from build123d import *

# Parameters (mm, degrees)
SKETCH1_R               = 8.895
BOSS_EXTRUDE1_DEPTH     = 25
CUT_EXTRUDE1_DEPTH      = 12.5
SKETCH3_R               = 1.984375
CUT_EXTRUDE2_DEPTH      = 9.895
CUT_EXTRUDE2_DEPTH_BACK = 9.895
CHAMFER1_SIZE           = 0.6


with BuildPart() as part:
    # Sketch1 → Boss-Extrude1 (new body)
    with BuildSketch(Plane(origin=(0, 0, 0), x_dir=(1, 0, 0), z_dir=(0, 1, 0))):
        Circle(SKETCH1_R)
    extrude(amount=-BOSS_EXTRUDE1_DEPTH)

    # Sketch2 → Cut-Extrude1 (cut)
    with BuildSketch(Plane.XZ.offset(25)):
        with BuildLine():
            Line((-6.83125, 1.984375), (-6.83125, -1.984375))
            Line((-6.83125, -1.984375), (-8.670829306, -1.984375))
            ThreePointArc((-8.670829306, -1.984375), (-8.895, 0), (-8.670829306, 1.984375))
            Line((-8.670829306, 1.984375), (-6.83125, 1.984375))
        make_face()
    cut_extrude1 = extrude(amount=-CUT_EXTRUDE1_DEPTH, mode=Mode.SUBTRACT)

    # Mirror1: Cut-Extrude1 across plane
    add(cut_extrude1.mirror(Plane(origin=(0, 0, 0), x_dir=(0, 0, 1), z_dir=(1, 0, 0))), mode=Mode.SUBTRACT)

    # Sketch3 → Cut-Extrude2 (cut, two sides)
    with BuildSketch(Plane(origin=(0, 0, 0), x_dir=(0, 0, -1), z_dir=(1, 0, 0))) as cut_extrude2_sk:
        with Locations((0, -12.5)):
            Circle(SKETCH3_R)
    extrude(amount=CUT_EXTRUDE2_DEPTH, mode=Mode.SUBTRACT)
    extrude(cut_extrude2_sk.sketch, amount=-CUT_EXTRUDE2_DEPTH_BACK, mode=Mode.SUBTRACT)

    # Sketch4 → Revolve1 (revolve)
    with BuildSketch(Plane.XY):
        with BuildLine():
            Line((0, 0), (0, 76.2))
            ThreePointArc((0, 76.2), (7.115842324, 38.394954096), (9.5, 0))
            Line((9.5, 0), (0, 0))
        make_face()
    revolve(axis=Axis((0, 0, 0), (0, 1, 0)))

    # Chamfer1
    chamfer1_edges = [part.edges().sort_by_distance(p)[0] for p in [
        (-8.895, 0, 0),
    ]]
    chamfer(chamfer1_edges, length=CHAMFER1_SIZE)


solid = part.part
Design review of the part built by this model. Coordinates are the model's own, in mm. A direction names the side the tool comes from. Give positions to 0.01 mm unless a question says otherwise; leave off trailing zeros. One line per question, with ' | ' between items. Start each with the question number.
(1) Draft analysis for pull direction Z (two halves, no side actions). For faces 3 (the face through (-6.831, -19, 0)), 4 (the face through (8.484, -12.629, -2.672)), 5 (the face through (0, -25, 0)), state which applies: +Z half, -Z half, draft (parallel to the pull), parting line (faces both ways), or undercut.
(2) For line 1 (Z direction, x = -5.75, y = -12.5); line 2 (Z direction, x = -6, y = -12.5); line 3 (X direction, y = 16, z = -6.5), list the stretches that pass through material, from the lowest coordinate up.
(3) Insertion check: P1, Ø4, axis at x = -4.5, y = -4, coming from the -Z side; P2, Ø1, axis at x = -6, y = 23, coming from the -Z side; P3, Ø5, axis at y = -12.5, z = 0, coming from the -X side (3 decimals); P4, Ø2, axis at y = 65, z = -5.5, coming from the -X side. Each pin has a flat end and moves straight along its axis. Give the tip position at first contact, or say it passes through.
(4) For faces 1 (the face through (6.831, -19, 0)), 2 (the face through (-8, -19, -1.984)), list the 3-axis set-ups (+Z, -Z, +X, -X, +Y, -Y) from which the entire face can be reached by the end or side of a thin tool; tool diameter is ignored.
The answers:
1) face 3: undercut | face 4: parting line | face 5: draft
2) line 1: z = -6.79 to -1.98, 1.98 to 6.79 | line 2: z = -6.57 to -1.98, 1.98 to 6.57 | line 3: x = -6.35 to 6.35
3) P1: stops at z = -8.54 | P2: stops at z = -6.67 | P3: stops at x = -8.895 | P4: passes through
4) face 1: +X, -Y | face 2: -X, -Y
